Read the model definition and answer for the solid it produces. Units are mm, in the model's axes. Face numbers are marked on the shaded views. Give positions to 0.01 mm unless a question says otherwise; leave off trailing zeros. Write each loop counter-clockwise with the first axis right and the second up, starting at its lowest first coordinate (ties: lowest second). Pieces come first, ordered by that corner, then holes. Notation, with made-up numbers: (72, 1) - (87, 1) arc R9 ccw to (87, 12) - close; hole circle Ø9 at (-28, -31). An arc over 180 degrees is marked (long way). Answer as CSV lines item,"result".
```python
from build123d import *

# Parameters (mm, degrees)
SKETCH1_W            = 388.7
SKETCH1_H            = 435.95
SKETCH1_W_2          = 45.6
SKETCH1_H_2          = 430.25
BOSS_EXTRUDE1_DEPTH  = 189
BOSS_EXTRUDE2_START  = -433.45
SKETCH2_W            = 388.7
SKETCH2_H            = 3.2
BOSS_EXTRUDE2_DEPTH  = 430.25
CUT_EXTRUDE1_DEPTH   = 25
BOSS_EXTRUDE4_DEPTH  = 3.2
BOSS_EXTRUDE5_DEPTH  = 3.2
BOSS_EXTRUDE6_REACH  = 791.664
CUT_EXTRUDE2_REACH   = 793.231
SKETCH11_W           = 52.59
SKETCH11_H           = 168.019571709
BOSS_EXTRUDE7_DEPTH  = 3.2
BOSS_EXTRUDE8_DEPTH  = 3.2
SKETCH14_W           = 388.7
SKETCH14_H           = 3.2
BOSS_EXTRUDE9_DEPTH  = 40
SKETCH15_W           = 388.7
SKETCH15_H           = 3.2
BOSS_EXTRUDE10_DEPTH = 40
SKETCH16_W           = 693.36
SKETCH16_H           = 3.2
BOSS_EXTRUDE11_DEPTH = 43.15
SKETCH17_W           = 693.36
SKETCH17_H           = 3.2
BOSS_EXTRUDE12_DEPTH = 43.15


with BuildPart() as part:
    # Sketch1 → Boss-Extrude1 (new body)
    with BuildSketch(Plane(origin=(0, 0, 0), x_dir=(1, 0, 0), z_dir=(0, 1, 0))):
        with Locations((191.15, 214.775)):
            Rectangle(SKETCH1_W, SKETCH1_H)
        with Locations((22.8, 215.125)):
            Rectangle(SKETCH1_W_2, SKETCH1_H_2, mode=Mode.SUBTRACT)
        with Locations((359.5, 215.125)):
            Rectangle(SKETCH1_W_2, SKETCH1_H_2, mode=Mode.SUBTRACT)
        with Locations((70.9, 215.125)):
            Rectangle(SKETCH1_W_2, SKETCH1_H_2, mode=Mode.SUBTRACT)
        with Locations((119, 215.125)):
            Rectangle(SKETCH1_W_2, SKETCH1_H_2, mode=Mode.SUBTRACT)
        with Locations((167.1, 215.125)):
            Rectangle(SKETCH1_W_2, SKETCH1_H_2, mode=Mode.SUBTRACT)
        with Locations((215.2, 215.125)):
            Rectangle(SKETCH1_W_2, SKETCH1_H_2, mode=Mode.SUBTRACT)
        with Locations((263.3, 215.125)):
            Rectangle(SKETCH1_W_2, SKETCH1_H_2, mode=Mode.SUBTRACT)
        with Locations((311.4, 215.125)):
            Rectangle(SKETCH1_W_2, SKETCH1_H_2, mode=Mode.SUBTRACT)
    extrude(amount=BOSS_EXTRUDE1_DEPTH)

    # Sketch2 → Boss-Extrude2 (add)
    with BuildSketch(Plane.XY.offset(3.2).offset(BOSS_EXTRUDE2_START)):
        with Locations((191.15, 1.6)):
            Rectangle(SKETCH2_W, SKETCH2_H)
    extrude(amount=BOSS_EXTRUDE2_DEPTH)

    # Sketch3 → Cut-Extrude1 (cut)
    with BuildSketch(Plane(origin=(0, 189, 0), x_dir=(1, 0, 0), z_dir=(0, 1, 0))):
        Polygon((0, 430.25), (0, 432.75), (382.3, 432.75), (382.3, 430.25), (336.7, 430.25), (336.7, 0), (334.2, 0), (334.2, 430.25), (288.6, 430.25), (288.6, 0), (286.1, 0), (286.1, 430.25), (240.5, 430.25), (240.5, 0), (238, 0), (238, 430.25), (192.4, 430.25), (192.4, 0), (189.9, 0), (189.9, 430.25), (144.3, 430.25), (144.3, 0), (141.8, 0), (141.8, 430.25), (96.2, 430.25), (96.2, 0), (93.7, 0), (93.7, 430.25), (48.1, 430.25), (48.1, 0), (45.6, 0), (45.6, 430.25), align=None)
    extrude(amount=-CUT_EXTRUDE1_DEPTH, mode=Mode.SUBTRACT)

    # Sketch4 → Boss-Extrude4 (add)
    with BuildSketch(Plane(origin=(385.5, 0, 0), x_dir=(0, 0, -1), z_dir=(1, 0, 0))):
        Polygon((432.75, 189), (662.75, 0), (432.75, 0), align=None)
    extrude(amount=-BOSS_EXTRUDE4_DEPTH)

    # Sketch7 → Boss-Extrude5 (add)
    with BuildSketch(Plane.ZY.offset(3.2)):
        Polygon((-432.75, 164), (-432.75, 189), (-662.75, 0), (-432.75, 0), align=None)
    extrude(amount=-BOSS_EXTRUDE5_DEPTH)

    # Sketch9 → Boss-Extrude6 (add, up to next)
    with BuildSketch(Plane(origin=(0, 0, 0), x_dir=(0, 0, -1), z_dir=(1, 0, 0)), mode=Mode.PRIVATE) as boss_extrude6_sk1:
        Polygon((662.75, 0), (658.855820106, 3.2), (432.75, 3.2), (432.75, 0), align=None)
    boss_extrude6_tool1 = extrude(boss_extrude6_sk1.sketch, amount=BOSS_EXTRUDE6_REACH, mode=Mode.PRIVATE) - part.part
    add(boss_extrude6_tool1.solids().sort_by_distance((0, 1.595446, -546.779226))[0])

    # Sketch11 → Cut-Extrude2 (cut, up to next)
    with BuildSketch(Plane(origin=(385.5, 0, 0), x_dir=(0, 0, -1), z_dir=(1, 0, 0)), mode=Mode.PRIVATE) as cut_extrude2_sk1:
        with Locations((636.455, 84.009785855)):
            Rectangle(SKETCH11_W, SKETCH11_H)
    cut_extrude2_tool1 = extrude(cut_extrude2_sk1.sketch, amount=-CUT_EXTRUDE2_REACH, mode=Mode.PRIVATE) & part.part
    add(cut_extrude2_tool1.solids().sort_by_distance((385.5, 84.009786, -636.455))[0], mode=Mode.SUBTRACT)

    # Sketch12 → Boss-Extrude7 (add)
    with BuildSketch(Plane(origin=(385.5, 0, 0), x_dir=(0, 0, -1), z_dir=(1, 0, 0))):
        Polygon((456.376412276, 189), (610.16, 62.630008348), (610.16, 43.21526087), (432.75, 189), align=None)
    extrude(amount=-BOSS_EXTRUDE7_DEPTH)

    # Sketch13 → Boss-Extrude8 (add)
    with BuildSketch(Plane.ZY.offset(3.2)):
        Polygon((-610.16, 62.630008348), (-610.16, 43.21526087), (-432.75, 189), (-456.376412276, 189), align=None)
    extrude(amount=-BOSS_EXTRUDE8_DEPTH)

    # Sketch14 → Boss-Extrude9 (add)
    with BuildSketch(Plane(origin=(0, 0, -610.16), x_dir=(-1, 0, 0), z_dir=(0, 0, -1))):
        with Locations((-191.15, 1.6)):
            Rectangle(SKETCH14_W, SKETCH14_H)
    extrude(amount=BOSS_EXTRUDE9_DEPTH)

    # Sketch15 → Boss-Extrude10 (add)
    with BuildSketch(Plane.XY.offset(3.2)):
        with Locations((191.15, 1.6)):
            Rectangle(SKETCH15_W, SKETCH15_H)
    extrude(amount=BOSS_EXTRUDE10_DEPTH)

    # Sketch16 → Boss-Extrude11 (add)
    with BuildSketch(Plane(origin=(385.5, 0, 0), x_dir=(0, 0, -1), z_dir=(1, 0, 0))):
        with Locations((303.48, 1.6)):
            Rectangle(SKETCH16_W, SKETCH16_H)
    extrude(amount=BOSS_EXTRUDE11_DEPTH)

    # Sketch17 → Boss-Extrude12 (add)
    with BuildSketch(Plane.ZY.offset(3.2)):
        with Locations((-303.48, 1.6)):
            Rectangle(SKETCH17_W, SKETCH17_H)
    extrude(amount=BOSS_EXTRUDE12_DEPTH)


solid = part.part
```
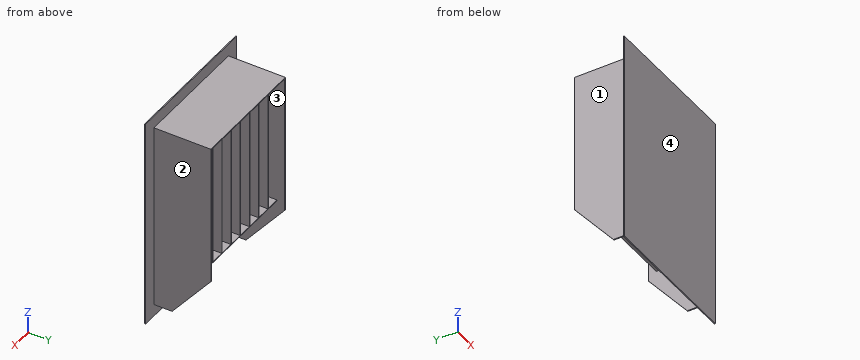
(1) A cutting plane is placed at B-B (y = 52). Count the separate pieces of the cut face and the enclosed holes in it, and give its area (3 significant figures).
Worked out:
separate pieces,"1"
enclosed holes,"8"
area,"13,600 mm^2"
(2) Each of these flat-tipped pins is pushed along its axis until it touches: P1, Ø12, axis at x = 25.5, z = -254.5, coming from the -Y side; P2, Ø4, axis at x = 294, z = -175.5, coming from the +Y side; P3, Ø1, axis at x = 97, y = 31, coming from the +Z side; P4, Ø3, axis at x = 244.5, y = 23, coming from the -Z side. Where does it stop, or does it pass through?
Worked out:
P1,"stops at y = 0"
P2,"stops at y = 3.2"
P3,"stops at z = 3.2"
P4,"stops at z = -432.75"
(3) The mould has two halves that part along X. Classify the marked faces 1, 2, 3 and 4: +X half, -X half, draft (parallel to the pull), parting line (faces both ways), or undercut.
Worked out:
face 1,"-X half"
face 2,"+X half"
face 3,"undercut"
face 4,"draft"
(4) A cutting plane is placed at C-C (z = -505.5). Write down the section's boundary in (x, y).
Worked out:
outline,"(-46.35, 0) - (428.65, 0) - (428.65, 3.2) - (385.5, 3.2) - (385.5, 148.63) - (382.3, 148.63) - (382.3, 3.2) - (0, 3.2) - (0, 148.63) - (-3.2, 148.63) - (-3.2, 3.2) - (-46.35, 3.2) - close"
(5) A cutting plane is placed at A-A (x = 103.5). Write down the section's boundary in (y, z), and give its area (3 significant figures).
Worked out:
outline,"(0, -650.16) - (3.2, -650.16) - (3.2, -432.75) - (164, -432.75) - (164, -430.25) - (3.2, -430.25) - (3.2, 0) - (189, 0) - (189, 3.2) - (3.2, 3.2) - (3.2, 43.2) - (0, 43.2) - close"
area,"3,220 mm^2"
(6) Find the intervals of material crossed by L1, parallel to Z at x = 333.5, y = 90.5; L2, parallel to X at y = 39.5, z = -513; L3, parallel to Y at x = 116, z = -311, in increasing order.
Worked out:
L1,"z = -432.75 to -430.25, 0 to 3.2"
L2,"x = -3.2 to 0, 382.3 to 385.5"
L3,"y = 0 to 3.2"
